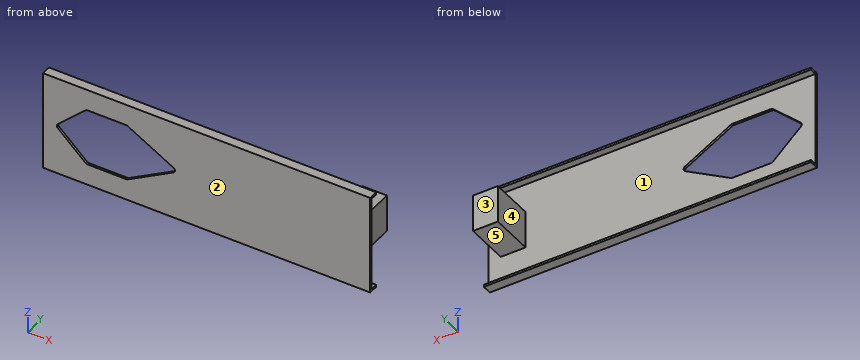
```python
from build123d import *

# Parameters (mm, degrees)
SKETCH1_W           = 669.925
SKETCH1_H           = 203.2
BOSS_EXTRUDE1_DEPTH = 4.6228
SKETCH2_W           = 669.925
SKETCH2_H           = 4.6228
BOSS_EXTRUDE2_DEPTH = 14.732
CUT_EXTRUDE1_DEPTH  = 5.6228
FILLET1_R           = 5.842
SKETCH4_W           = 50.8
SKETCH4_H           = 76.2
BOSS_EXTRUDE3_DEPTH = 88.9


with BuildPart() as part:
    # Sketch1 → Boss-Extrude1 (new body)
    with BuildSketch(Plane(origin=(0, 0, 0), x_dir=(1, 0, 0), z_dir=(0, 1, 0))):
        with Locations((334.9625, 101.6)):
            Rectangle(SKETCH1_W, SKETCH1_H)
    extrude(amount=BOSS_EXTRUDE1_DEPTH)

    # Sketch2 → Boss-Extrude2 (add)
    with BuildSketch(Plane(origin=(0, 4.6228, 0), x_dir=(1, 0, 0), z_dir=(0, 1, 0))):
        with Locations((334.9625, 2.3114)):
            Rectangle(SKETCH2_W, SKETCH2_H)
        with Locations((334.9625, 200.8886)):
            Rectangle(SKETCH2_W, SKETCH2_H)
    extrude(amount=BOSS_EXTRUDE2_DEPTH)

    # Sketch3 → Cut-Extrude1 (cut, through all)
    with BuildSketch(Plane(origin=(0, 4.6228, 0), x_dir=(1, 0, 0), z_dir=(0, 1, 0))):
        Polygon((171.958, 43.4975), (88.9, 43.4975), (25.4, 101.6), (88.9, 159.7025), (171.958, 159.7025), (276.225, 101.3968), align=None)
    extrude(amount=-CUT_EXTRUDE1_DEPTH, mode=Mode.SUBTRACT)

    # Fillet1
    fillet1_edges = [part.edges().sort_by_distance(p)[0] for p in [
        (171.958, 2.3114, -159.7025),
        (276.225, 2.3114, -101.3968),
        (171.958, 2.3114, -43.4975),
        (88.9, 2.3114, -43.4975),
        (25.4, 2.3114, -101.6),
        (88.9, 2.3114, -159.7025),
    ]]
    fillet(fillet1_edges, radius=FILLET1_R)

    # Sketch4 → Boss-Extrude3 (add)
    with BuildSketch(Plane(origin=(0, 4.6228, 0), x_dir=(1, 0, 0), z_dir=(0, 1, 0))):
        with Locations((619.125, 101.6)):
            Rectangle(SKETCH4_W, SKETCH4_H)
    extrude(amount=BOSS_EXTRUDE3_DEPTH)


solid = part.part
```
Build history of the part. All positions in model axes, mm. Face numbers are marked on the shaded views. A direction names the side the tool comes from. Round coordinates to 2 decimals unless told otherwise and drop trailing zeros. Loops run counter-clockwise (first coordinate to the right, second up) from the corner with the lowest first, then second, coordinate; pieces in that order, holes last.
Item 1: Drill centre lines: line 1 along Z through (x, y) = (92, 15); line 2 along X through (y, z) = (44, -114) (3 decimals); line 3 along Y through (x, z) = (516.5, -121.5). Where is each one in solid material? Low to high.
Item 2: Saw through at B-B (z = -148.5). List the corners of the cut face in (x, y) (3 decimals).
Item 3: Two-plate mould, pull along Z, no slides. Class the marked faces 1 and 2: released by +Z, released by -Z, zero draft, split by the parting line, or undercut.
Item 4: Which spindle directions (+Z, -Z, +X, -X, +Y, -Y) get a long thin tool onto all of the face, cutting with end or side? Do the marked faces 3, 4 and 5. Say none if no direction does.
Item 5: Pin check, flat tips, straight feed: P1, Ø1.4, axis at x = 140.5, y = 1.5, coming from the +Z side; P2, Ø15, axis at x = 624, y = 58.5, coming from the +Z side; P3, Ø3.5, axis at x = 366.5, z = -3, coming from the +Y side; P4, Ø6, axis at x = 594, z = -46.5, coming from the +Y side. Stop position of each tip, or through.
Item 6: Saw through at D-D (y = 80). List the corners of the cut face in (x, z) (3 decimals).
Item 7: Saw through at A-A (x = 126). List the corners of the cut face in (y, z), then the cut area to 3 significant figures.
Item 8: Saw through at C-C (x = 506). List the corners of the cut face in (y, z), then the cut area to 3 significant figures.
Worked answers:
1. line 1: z = -203.2 to -198.58, -4.62 to 0
1. line 2: x = 593.725 to 644.525
1. line 3: y = 0 to 4.62
2. outline: (0, 0) - (76.657, 0) - (76.657, 4.623) - (0, 4.623) - close; (191.991, 0) - (669.925, 0) - (669.925, 4.623) - (191.991, 4.623) - close
3. face 1: undercut
3. face 2: zero draft
4. face 3: +Z, -Z, +X, -X, +Y
4. face 4: -X, +Y
4. face 5: +X, -X, +Y
5. P1: stops at z = 0
5. P2: stops at z = -63.5
5. P3: stops at y = 19.35
5. P4: stops at y = 4.62
6. outline: (593.725, -139.7) - (644.525, -139.7) - (644.525, -63.5) - (593.725, -63.5) - close
7. outline: (0, -203.2) - (19.35, -203.2) - (19.35, -198.58) - (4.62, -198.58) - (4.62, -159.7) - (0, -159.7) - close; (0, -43.5) - (4.62, -43.5) - (4.62, -4.62) - (19.35, -4.62) - (19.35, 0) - (0, 0) - close
7. area: 538 mm2
8. outline: (0, -203.2) - (19.35, -203.2) - (19.35, -198.58) - (4.62, -198.58) - (4.62, -4.62) - (19.35, -4.62) - (19.35, 0) - (0, 0) - close
8. area: 1,080 mm2
